Verification items for the finished model (mm, model axes). Face numbers are marked on the shaded views. A direction names the side the tool comes from. Coordinates: 2 decimals unless noted, no trailing zeros. Write each loop counter-clockwise with the first axis right and the second up, starting at its lowest first coordinate (ties: lowest second). Pieces come first, ordered by that corner, then holes. Notation, with made-up numbers: (-38.75, -23) - (-31.75, -23) arc R31 ccw to (-31.75, 15) - close; hole circle Ø9 at (60, 7). An arc over 180 degrees is marked (long way). Use one line per item in the form item = value. Start each with the question number.
(1) Sectioned sample at B-B (y = -8). Record the cut outline in (x, z).
(2) Sectioned sample at A-A (y = -66). Record the cut outline in (x, z).
(3) Gauge pin test, flat ends, axial feed: pin 1 Ø6.5 at (y, z) = (-15.5, -45.5) entering from +X; pin 2 Ø5 at (x, z) = (20.5, -14) entering from +Y; pin 3 Ø6.5 at (y, z) = (4, 2) entering from -X. Record the tip position at first contact, or that the pin passes through.
(4) Tool access check on the marked faces 1 and 2. Record the directions out of +Z, -Z, +X, -X, +Y, -Y that give a thin tool (end or side, any length) a straight path to the whole face; none if there is none.
(5) Mould release check, pull along Z, two halves, no side actions. Record for the marked faces 3, 4, 5 and 6: released by +Z, released by -Z, zero draft, split by the parting line, or undercut.
(6) Sectioned sample at C-C (x = 0). Record the cut outline in (y, z), and give its area (3 significant figures).
(7) Material ranges on line 1 (Z direction, x = 14, y = -61); line 2 (Y direction, x = 3, z = -38); line 3 (X direction, y = -11, z = 4), recorded low to high. Write a range as [from, to].
(8) Sectioned sample at D-D (x = 26). Record the cut outline in (y, z).
Autodesk Inventor part; units mm, degrees
ref_plane "YZ Plane" through (0, 0, 0) normal (1, 0, 0) x (0, 1, 0)
ref_plane "XZ Plane" through (0, 0, 0) normal (0, 1, 0) x (-1, 0, 0)
ref_plane "XY Plane" through (0, 0, 0) normal (0, 0, 1) x (1, 0, 0)
sketch "스케치1" plane through (0, 0, 0) normal (0, 0, 1) x (1, 0, 0)
  circle A0 centre (0, 8) radius 1.05
  line L0 (6.1695, 0) -> (-5.6569, 0)
  circle A1 centre (0, 0) radius 11
  line L1 (11, -20) -> (31, -20)
  line L2 (11, 0) -> (11, -20)
  arc A2 (11, 0) -> (7.5778, 7.9735) centre (0, 0) ccw
  arc A3 (-7.5778, 7.9735) -> (-11, 0) centre (0, 0) ccw
  line L3 (-11, -40) -> (-11, 0)
  line L4 (31, -40) -> (-11, -40)
  line L5 (31, -20) -> (31, -40)
  circle A4 centre (5.6569, 5.6569) radius 1.2
  circle A5 centre (-8, 0) radius 1.2
  circle A6 centre (-5.6569, 5.6569) radius 1.2
  circle A7 centre (-5.6569, -5.6569) radius 1.2
  circle A8 centre (5.6569, -5.6569) radius 1.2
  circle A9 centre (0, -8) radius 1.2
  circle A10 centre (8, 0) radius 1.2
  arc A11 (-10.0222, 4.5338) -> (10.0222, 4.5338) centre (0, 0) ccw
  arc A12 (-4.2, 0) -> (4.2, 0) centre (0, 0) ccw
  line L6 (4.2, 0) -> (-4.2, 0)
  line L7 (-4.2, 0) -> (-4.2, 6.5238)
  line L8 (-4.2, 13.5959) -> (4.2, 13.5959)
  line L9 (4.2, 6.5238) -> (4.2, 0)
  arc A13 (-7.5778, 7.9735) -> (7.5778, 7.9735) centre (0, 0) ccw
  arc A14 (7.5778, 7.9735) -> (4.2, 6.5238) centre (6.2, 6.5238) ccw
  arc A15 (-4.2, 6.5238) -> (-7.5778, 7.9735) centre (-6.2, 6.5238) ccw
  point P0 (-6.2, 0)
  point P1 (4.2, 10.1666)
  point P2 (-4.2, 10.1666)
  point P3 (-7.5778, 7.9735)
  point P4 (7.5778, 7.9735)
  dimension "d20" = 2
extrude "돌출1" add sketch "스케치1" along normal blind 6 contours L9 A14 A1 A15 L7 A12
sketch "스케치3" plane through (0, 0, 6) normal (0, 0, 1) x (1, 0, 0)
  line L0 (31, -40) -> (31, -20)
  line L1 (11, -20) -> (31, -20)
  line L2 (31, -20) -> (31, -40)
  line L3 (31, -40) -> (11, -40)
  line L4 (11, -40) -> (11, -20)
  arc A0 (-7.5778, 7.9735) -> (7.5778, 7.9735) centre (0, 0) ccw
  circle A1 centre (-8, 0) radius 1.2
  circle A2 centre (-5.6569, -5.6569) radius 1.2
  circle A3 centre (5.6569, -5.6569) radius 1.2
  circle A4 centre (0, -8) radius 1.2
  circle A5 centre (8, 0) radius 1.2
  line L5 (11, -40) -> (-11, -40)
  line L6 (-11, -40) -> (-11, -80)
  line L7 (-11, -80) -> (11, -80)
  line L8 (11, -80) -> (11, -40)
  line L9 (-11, -80) -> (29, -80)
  line L10 (29, -80) -> (29, -60)
  line L11 (29, -60) -> (-11, -60)
  line L12 (-11, -60) -> (-11, -80)
  line L13 (-11, -40) -> (11, -40)
  line L14 (11, -40) -> (11, 0)
  line L15 (11, 0) -> (-11, 0)
  line L16 (-11, 0) -> (-11, -40)
  arc A6 (7.5778, 7.9735) -> (4.2, 6.5238) centre (6.2, 6.5238) ccw
  line L17 (4.2, 6.5238) -> (4.2, 0)
  arc A7 (-4.2, 0) -> (4.2, 0) centre (0, 0) ccw
  line L18 (-4.2, 0) -> (-4.2, 6.5238)
  arc A8 (-4.2, 6.5238) -> (-7.5778, 7.9735) centre (-6.2, 6.5238) ccw
  point P0 (11, -60)
  dimension "d4" = 40
extrude "돌출2" add sketch "스케치3" against normal blind 6 contours L5 L16 A0 L14 L4 | L8 L11 L6 L5 | L11 L10 L9 L8 | L8 L7 L6 L11
sketch "스케치4" plane through (0, 0, 0) normal (0, 0, -1) x (-1, 0, 0)
  line L0 (11, 0) -> (11, -80)
  line L1 (-29, -60) -> (-29, -80)
  line L2 (11, -80) -> (-29, -80)
  line L3 (-29, -80) -> (-29, -60)
  line L4 (-29, -60) -> (11, -60)
  line L5 (11, -60) -> (11, -80)
  line L6 (11, -80) -> (-29, -80)
  line L7 (-29, -80) -> (-29, -74)
  line L8 (-29, -74) -> (11, -74)
  line L9 (11, -74) -> (11, -80)
  point P0 (0, 0)
  dimension "d7" = 6
extrude "돌출3" add sketch "스케치4" along normal blind 41.2 contours L0 L2 L1 L8
sketch "스케치5" plane through (0, 0, -41.2) normal (0, 0, -1) x (-1, 0, 0)
  circle A0 centre (0, 0) radius 11
  circle A1 centre (5.6569, -5.6569) radius 1.15
  circle A2 centre (8, 0) radius 1.15
  circle A3 centre (5.6569, 5.6569) radius 1.15
  circle A4 centre (0, 8) radius 1.15
  circle A5 centre (-5.6569, 5.6569) radius 1.15
  circle A6 centre (-8, 0) radius 1.15
  circle A7 centre (-5.6569, -5.6569) radius 1.15
  circle A8 centre (0, -8) radius 1.15
  line L0 (-11, 0) -> (-11, -60)
  line L1 (11, 0) -> (11, -80)
  line L2 (-11, 0) -> (11, 0)
  line L3 (11, 0) -> (11, -80)
  line L4 (11, -80) -> (-11, -80)
  line L5 (-11, -80) -> (-11, 0)
  line L6 (-29, -80) -> (-29, -60)
  line L7 (-29, -80) -> (-11, -80)
  line L8 (-11, -80) -> (-11, -60)
  line L9 (-11, -60) -> (-29, -60)
  line L10 (-29, -60) -> (-29, -80)
  line L11 (6.2, 0) -> (-6.2, 0)
  line L12 (-6.2, 15) -> (6.2, 15)
  arc A9 (-10.0222, 4.5338) -> (10.0222, 4.5338) centre (0, 0) ccw
  arc A10 (11, 0) -> (7.5778, 7.9735) centre (0, 0) ccw
  line L13 (11, 0) -> (11, -80)
  line L14 (11, -80) -> (-29, -80)
  line L15 (-29, -80) -> (-29, -60)
  line L16 (-29, -60) -> (-11, -60)
  line L17 (-11, -60) -> (-11, 0)
  arc A11 (-7.5778, 7.9735) -> (-11, 0) centre (0, 0) ccw
  arc A12 (-4.2, 6.5238) -> (-7.5778, 7.9735) centre (-6.2, 6.5238) ccw
  line L18 (-4.2, 6.5238) -> (-4.2, 0)
  arc A13 (-4.2, 0) -> (4.2, 0) centre (0, 0) ccw
  line L19 (4.2, 0) -> (4.2, 6.5238)
  arc A14 (7.5778, 7.9735) -> (4.2, 6.5238) centre (6.2, 6.5238) ccw
  circle A15 centre (-8, 0) radius 1.2
  circle A16 centre (0, -8) radius 1.2
  circle A17 centre (-5.6569, -5.6569) radius 1.2
  circle A18 centre (5.6569, -5.6569) radius 1.2
  circle A19 centre (5.6569, 5.6569) radius 1.2
  circle A20 centre (8, 0) radius 1.2
  circle A21 centre (-5.6569, 5.6569) radius 1.2
  circle A22 centre (5.6569, 5.6569) radius 1.1
  circle A23 centre (0, 8) radius 1.1
  circle A24 centre (-5.6569, 5.6569) radius 1.1
  circle A25 centre (-8, 0) radius 1.1
  circle A26 centre (-5.6569, -5.6569) radius 1.1
  circle A27 centre (0, -8) radius 1.1
  circle A28 centre (5.6569, -5.6569) radius 1.1
  circle A29 centre (8, 0) radius 1.1
  point P0 (0, 0)
  point P1 (6.2, 9.0863)
  point P2 (-6.2, 9.0863)
  point P3 (11, 0)
  point P4 (9.2, 0)
  point P5 (6.8, 0)
  point P6 (6.85, 0)
  point P7 (9.15, 0)
  point P8 (7.5778, 7.9735)
  point P9 (-7.5778, 7.9735)
  point P10 (6.9, 0)
  point P11 (9.1, 0)
  point P12 (-6.9, 0)
  point P13 (-9.1, 0)
  point P14 (-9.15, 0)
  point P15 (-6.85, 0)
  dimension "d13" = 360
  dimension "d21" = 2.2
  dimension "d24" = 360
extrude "돌출4" add sketch "스케치5" along normal blind 6 contours L2 A20 L19 A14 A0 | L1 L4 L5 L0 A0 | A0 L2 A15 A13 A20 | A0 A12 L18 L2 A15 | L2 A2 A20 | L5 L7 L6 L9 | A15 L2 A6 | L2 A6 A15 | L2 A29 A2 | L2 A25 A6 | A6 L2 A25 | A1 | A3 | A5 | A7 | A8 | A16 | A17 | A18 | A19 | A21 picked at (7.9538, 1.1747) picked at (6.8885, 0.1795)
properties part number "부품56" material "PMMA 플라스틱"
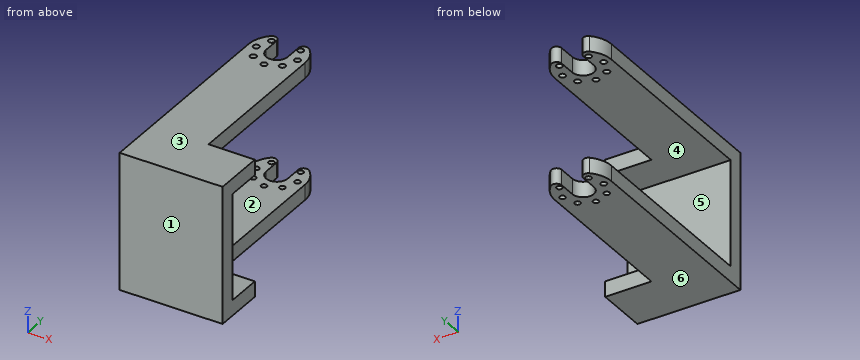
Answers below:
q1.outline = (-11, -47.2) - (-1.1, -47.2) - (-1.1, -41.2) - (-11, -41.2) - close; (-11, 0) - (-1.2, 0) - (-1.2, 6) - (-11, 6) - close; (1.1, -47.2) - (11, -47.2) - (11, -41.2) - (1.1, -41.2) - close; (1.2, 0) - (11, 0) - (11, 6) - (1.2, 6) - close
q2.outline = (-11, -47.2) - (29, -47.2) - (29, -41.2) - (-11, -41.2) - close; (-11, 0) - (29, 0) - (29, 6) - (-11, 6) - close
q3.pin_1 = 11
q3.pin_2 = -74
q3.pin_3 = -10.97
q4.face_1 = +Z, -Z, +X, -X, -Y
q4.face_2 = +X, -X, +Y
q5.face_3 = released by +Z
q5.face_4 = undercut
q5.face_5 = undercut
q5.face_6 = released by -Z
q6.outline = (-80, -47.2) - (-9.1, -47.2) - (-9.1, -41.2) - (-74, -41.2) - (-74, 0) - (-9.2, 0) - (-9.2, 6) - (-80, 6) - close; (-6.9, -47.2) - (-4.2, -47.2) - (-4.2, -41.2) - (-6.9, -41.2) - close; (-6.8, 0) - (-4.2, 0) - (-4.2, 6) - (-6.8, 6) - close
q6.area = 1,130 mm2
q7.line_1 = [-47.2, -41.2], [0, 6]
q7.line_2 = [-80, -74]
q7.line_3 = [-11, 11]
q8.outline = (-80, -47.2) - (-60, -47.2) - (-60, -41.2) - (-74, -41.2) - (-74, 0) - (-60, 0) - (-60, 6) - (-80, 6) - close
